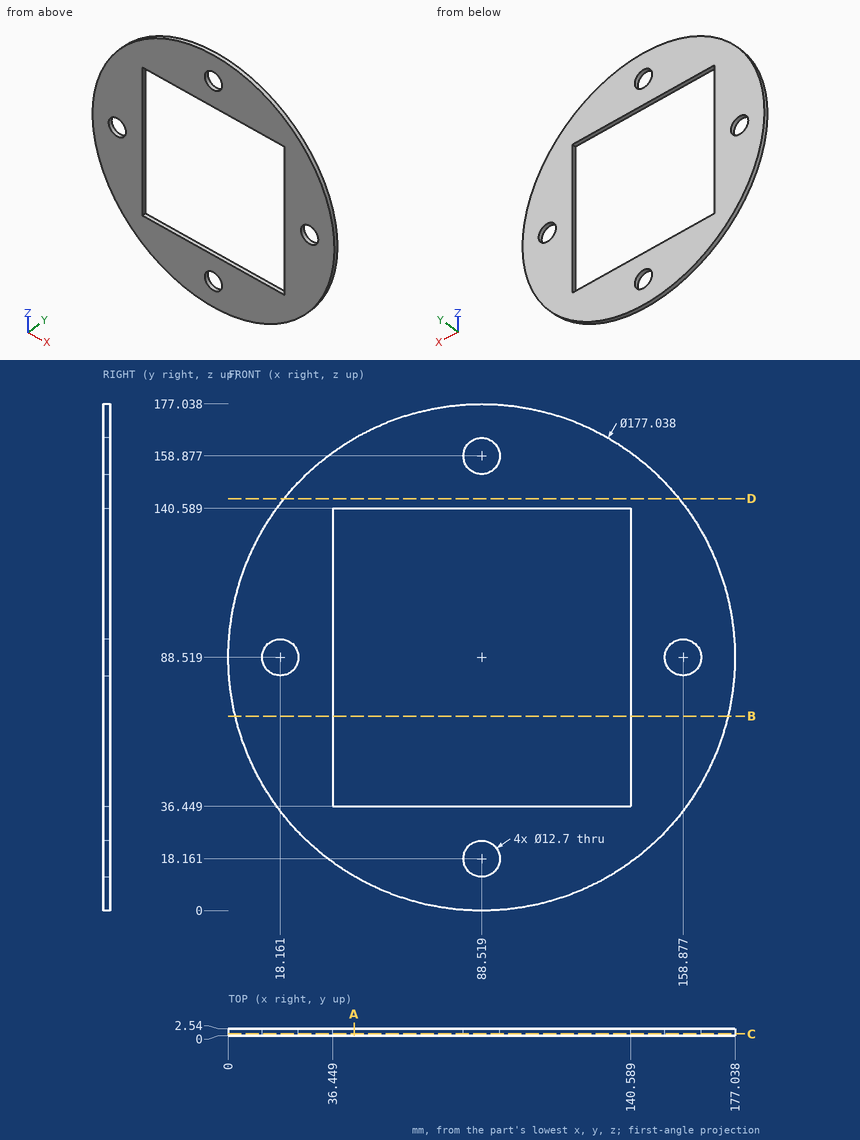
The drawing under review shows one solid part. Ordinate dimensions are in mm from its lowest x, y, z. Round coordinates to 2 decimals unless told otherwise and drop trailing zeros. Write each loop counter-clockwise with the first axis right and the second up, starting at its lowest first coordinate (ties: lowest second). Pieces come first, ordered by that corner, then holes. Notation, with made-up numbers: M 17,18.25 L 23,18.25 A20 ccw 23,44.25 Z; hole C -29.5,25 d2. An arc over 180 degrees is marked long. One line per item, written item: value. Start each with the question number.
(1) We need section A-A (x = 44). Give the boundary of the cut face in (y, z).
(2) We need section B-B (z = 68). Give the boundary of the cut face in (x, y), and give its area (3 significant figures).
(3) We need section C-C (y = 0.7). Give the boundary of the cut face in (x, z), and give its area (3 significant figures).
(4) Wall thickness on line 1 (Z direction, x = 48, y = 1.7); line 2 (Z direction, x = 84, y = 0.55); line 3 (X direction, y = 0.2, z = 120): over which ranges is each line inside the solid? List them lowest first.
(5) Insertion check: pin 1 (1 mm diameter, centred on x = 63, y = 0.5, fed in from +Z); pin 2 (0.8 mm diameter, centred on x = 104.5, y = 1, fed in from -Z); pin 3 (1.3 mm diameter, centred on x = 98, y = 1.5, fed in from +Z). Each pin has a flat end and moves straight along its axis. Give the tip position at first contact, or say it passes through.
(6) We need section D-D (z = 144). Give the boundary of the cut face in (x, y), and give its area (3 significant figures).
Result:
1. outline: M 0,12.01 L 2.54,12.01 L 2.54,36.45 L 0,36.45 Z; M 0,140.59 L 2.54,140.59 L 2.54,165.03 L 0,165.03 Z
2. outline: M 2.41,0 L 36.45,0 L 36.45,2.54 L 2.41,2.54 Z; M 140.59,0 L 174.63,0 L 174.63,2.54 L 140.59,2.54 Z
2. area: 173 mm²
3. outline: C 88.52,88.52 d177.04; hole C 18.16,88.52 d12.7; hole M 36.45,36.45 L 140.59,36.45 L 140.59,140.59 L 36.45,140.59 Z; hole C 88.52,18.16 d12.7; hole C 88.52,158.88 d12.7; hole C 158.88,88.52 d12.7
3. area: 13,300 mm²
4. line 1: 9.82 to 36.45, 140.59 to 167.22
4. line 2: 0.12 to 13.7, 22.62 to 36.45, 140.59 to 154.42, 163.34 to 176.92
4. line 3: 5.79 to 36.45, 140.59 to 171.25
5. pin 1: z = 173.43
5. pin 2: z = 1.38
5. pin 3: z = 176.6
6. outline: M 19.54,0 L 157.49,0 L 157.49,2.54 L 19.54,2.54 Z
6. area: 350 mm²
